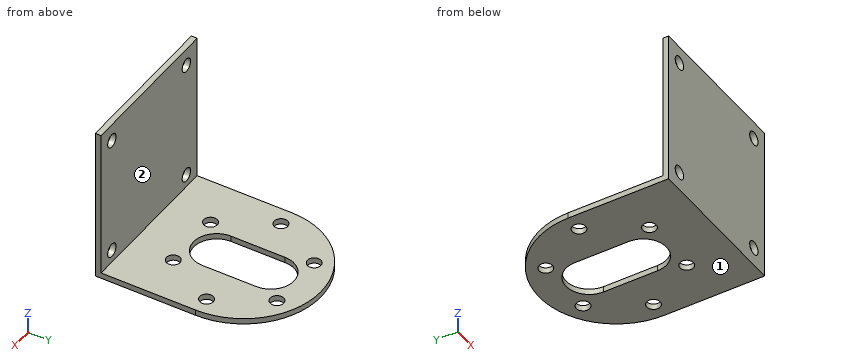
```python
from build123d import *

# Parameters (mm, degrees)
SKETCH1_R           = 1.75
BOSS_EXTRUDE1_DEPTH = 1.5
SKETCH2_W           = 40
SKETCH2_H           = 40.4
SKETCH2_R           = 1.75
BOSS_EXTRUDE2_DEPTH = 1.5


with BuildPart() as part:
    # Sketch1 → Boss-Extrude1 (new body)
    # profile 1 of 2: a face of its own
    with BuildSketch(Plane.XY):
        with BuildLine():
            Line((0, 26), (0, 0))
            Line((0, 0), (40, 0))
            Line((40, 0), (40, 26))
            Line((40, 26), (37.25, 26))
            ThreePointArc((37.25, 26), (35.5, 24.25), (33.75, 26))
            Line((33.75, 26), (26, 26))
            Line((26, 26), (26, 19))
            ThreePointArc((26, 19), (20, 13), (14, 19))
            Line((14, 19), (14, 26))
            Line((14, 26), (6.25, 26))
            ThreePointArc((6.25, 26), (4.5, 24.25), (2.75, 26))
            Line((2.75, 26), (0, 26))
        make_face()
        with Locations((12.25, 12.576606241)):
            Circle(SKETCH1_R, mode=Mode.SUBTRACT)
        with Locations((27.75, 12.576606241)):
            Circle(SKETCH1_R, mode=Mode.SUBTRACT)
    # profile 2 of 2: a face of its own
    with BuildSketch(Plane.XY):
        with BuildLine():
            ThreePointArc((40, 26), (20, 46), (0, 26))
            Line((0, 26), (2.75, 26))
            ThreePointArc((2.75, 26), (4.5, 27.75), (6.25, 26))
            Line((6.25, 26), (14, 26))
            Line((14, 26), (14, 33))
            ThreePointArc((14, 33), (20, 39), (26, 33))
            Line((26, 33), (26, 26))
            Line((26, 26), (33.75, 26))
            ThreePointArc((33.75, 26), (35.5, 27.75), (37.25, 26))
            Line((37.25, 26), (40, 26))
        make_face()
        with Locations((12.25, 39.423393759)):
            Circle(SKETCH1_R, mode=Mode.SUBTRACT)
        with Locations((27.75, 39.423393759)):
            Circle(SKETCH1_R, mode=Mode.SUBTRACT)
    extrude(amount=BOSS_EXTRUDE1_DEPTH)

    # Sketch2 → Boss-Extrude2 (add)
    with BuildSketch(Plane.XZ):
        with Locations((20, 20.2)):
            Rectangle(SKETCH2_W, SKETCH2_H)
        with Locations(Location((4.5, 35.855, 0), (0, 0, 270))):
            Circle(SKETCH2_R, mode=Mode.SUBTRACT)
        with Locations(Location((35.5, 35.855, 0), (0, 0, 270))):
            Circle(SKETCH2_R, mode=Mode.SUBTRACT)
        with Locations(Location((35.5, 4.855, 0), (0, 0, 270))):
            Circle(SKETCH2_R, mode=Mode.SUBTRACT)
        with Locations(Location((4.5, 4.855, 0), (0, 0, 270))):
            Circle(SKETCH2_R, mode=Mode.SUBTRACT)
    extrude(amount=-BOSS_EXTRUDE2_DEPTH)


solid = part.part
```
For this review, take the finished solid that the model builds, in its own axes (mm). Face numbers are marked on the shaded views. A direction names the side the tool comes from. Coordinates: 2 decimals unless noted, no trailing zeros. Loops run counter-clockwise (first coordinate to the right, second up) from the corner with the lowest first, then second, coordinate; pieces in that order, holes last. Notation, with made-up numbers: (28, -20) - (78, -20) arc R26 ccw to (78, 1) - close; hole circle Ø10 at (64.25, -2). An arc over 180 degrees is marked (long way). Use one line per item in the form item = value. Start each with the question number.
1) Take a section at D-D (x = 4.5). State the section outline as (y, z) points (3 decimals), plus the area to 3 significant figures.
2) For pin 1 (4 mm diameter, centred on x = 12.25, y = 12.58, fed in from +Z); pin 2 (1 mm diameter, centred on x = 27.5, z = 16, fed in from +Y); pin 3 (2 mm diameter, centred on x = 35.5, z = 35.855, fed in from -Y); pin 4 (1.6 mm diameter, centred on y = 27.5, z = 0.5, fed in from -X), all flat-tipped, find the tip position at first contact; note any pin that passes through.
3) Take a section at B-B (y = 32). State the section outline as (x, z) points.
4) Take a section at C-C (x = 27.75). State the section outline as (y, z) points.
5) For the marked faces 1 and 2, list the 3-axis set-ups (+Z, -Z, +X, -X, +Y, -Y) from which the entire face can be reached by the end or side of a thin tool; tool diameter is ignored.
6) To check wall thickness, follow probe 1 along Y at (x, z) = (12.25, 1.05); probe 2 along Z at (x, y) = (4, 1); probe 3 along Y at (x, z) = (21.5, 11.5). State the ranges of each line that lie inside material, in increasing order. Write a range as from..to.
7) Take a section at A-A (x = 20). State the section outline as (y, z) points.
From the geometry:
q1.outline = (0, 0) - (24.25, 0) - (24.25, 1.5) - (1.5, 1.5) - (1.5, 3.105) - (0, 3.105) - close; (0, 6.605) - (1.5, 6.605) - (1.5, 34.105) - (0, 34.105) - close; (0, 37.605) - (1.5, 37.605) - (1.5, 40.4) - (0, 40.4) - close; (27.75, 0) - (38.639, 0) - (38.639, 1.5) - (27.75, 1.5) - close
q1.area = 101 mm2
q2.pin_1 = 1.5
q2.pin_2 = 1.5
q2.pin_3 = through
q2.pin_4 = 0.01
q3.outline = (0.92, 0) - (14, 0) - (14, 1.5) - (0.92, 1.5) - close; (26, 0) - (39.08, 0) - (39.08, 1.5) - (26, 1.5) - close
q4.outline = (0, 0) - (10.83, 0) - (10.83, 1.5) - (1.5, 1.5) - (1.5, 40.4) - (0, 40.4) - close; (14.33, 0) - (37.67, 0) - (37.67, 1.5) - (14.33, 1.5) - close; (41.17, 0) - (44.44, 0) - (44.44, 1.5) - (41.17, 1.5) - close
q5.face_1 = -Z, +X, -X, +Y, -Y
q5.face_2 = +Z, +X, -X, +Y
q6.probe_1 = 0..10.83, 14.33..37.67, 41.17..44.44
q6.probe_2 = 0..3.18, 6.53..34.18, 37.53..40.4
q6.probe_3 = 0..1.5
q7.outline = (0, 0) - (13, 0) - (13, 1.5) - (1.5, 1.5) - (1.5, 40.4) - (0, 40.4) - close; (39, 0) - (46, 0) - (46, 1.5) - (39, 1.5) - close
